Read the model definition and answer for the solid it produces. Units are mm, in the model's axes. Face numbers are marked on the shaded views. A direction names the side the tool comes from. Round coordinates to 2 decimals unless told otherwise and drop trailing zeros. Order: outer loops, then holes, each group sorted by start corner. A loop starts at its lowest first (then second) coordinate and runs counter-clockwise, first axis right, second up. Notation, with made-up numbers: (80, 66.5) - (89, 66.5) arc R20 ccw to (89, 97.5) - close; hole circle Ø11 at (64.5, 70). An arc over 180 degrees is marked (long way). Answer as a JSON object with one key per item and string values. Group by question number.
Q1. Given pin 1 Ø4 at (y, z) = (-4.5, 23) entering from -X; pin 2 Ø1.5 at (y, z) = (-1, -26.5) entering from -X, each flat-ended and moving along its own axis, determine where each tip first touches the part or whether it passes through.
Q2. A cutting plane is placed at C-C on x = -47. Determine the outline of the cut face in (y, z), and give its area (3 significant figures).
Q3. Consider line 1 (X direction, y = -10.5, z = 18.5); line 2 (Z direction, x = -46, y = -1); line 3 (Z direction, x = -42.5, y = -5.5). Determine where each line is inside the solid, lowest interval first.
Q4. The mould has two halves that part along Z. Classify the marked faces 3, 4, 5 and 6: pulls with the +Z half, pulls with the -Z half, needs draft (parallel to the pull), parting line crosses it, or undercut.
Q5. A cutting plane is placed at B-B on y = -10.5. Count the separate pieces of the cut face and the enclosed holes in it, and give its area (3 significant figures).
Q6. A tool of negligible diameter and unlimited length cuts with its end or side. For the marked faces 1 and 2, from which of +Z, -Z, +X, -X, +Y, -Y can it reach the whole face along a straight path? Write none if from no direction.
Q7. A cutting plane is placed at A-A on z = 4. Determine the outline of the cut face in (x, y), and give its area (3 significant figures).
Q8. A cutting plane is placed at D-D on z = 13.5. Determine the outline of the cut face in (x, y).
```python
from build123d import *

# Parameters (mm, degrees)
F0_W     = 115
F0_H     = 70
F1_DEPTH = 12
F2_W     = 4.25
F2_H     = 5
F2_W_2   = 4.2500000007
F3_DEPTH = 25
F4_R     = 3.25
F5_DEPTH = 25
F6_R     = 15


with BuildPart() as f1:
    # F0 (on Front) → F1 (new body)
    with BuildSketch(Plane.XZ):
        Rectangle(F0_W, F0_H)
    extrude(amount=F1_DEPTH)

    # F2 (on face) → F3 (cut)
    with BuildSketch(Plane.XZ.offset(12)):
        with BuildLine():
            Line((-40.75, 16.25), (-40.75, 21.25))
            ThreePointArc((-40.75, 21.25), (-44.9763637107, 25.4999342731), (-49.2497370945, 21.2972718474))
            Line((-49.2497370945, 21.2972718474), (-49.2497419962, 21.2031708885))
            Line((-49.2497419962, 21.2031708885), (-49.2499999942, 16.2502213815))
            ThreePointArc((-49.2499999942, 16.2502213815), (-48.0052820892, 13.2448744512), (-45, 12))
            Line((-45, 12), (-45, 16.25))
            Line((-45, 16.25), (-40.75, 16.25))
        make_face()
        with BuildLine():
            ThreePointArc((49.2497370945, 21.2972718474), (44.9763637107, 25.4999342731), (40.75, 21.25))
            Line((40.75, 21.25), (40.75, 16.25))
            ThreePointArc((40.75, 16.25), (41.99479618, 19.25520382), (45, 20.5))
            ThreePointArc((45, 20.5), (46.9284060776, 20.0373143519), (48.4369317712, 18.75))
            ThreePointArc((48.4369317712, 18.75), (49.041590439, 17.5645519096), (49.2499999942, 16.2502213815))
            Line((49.2499999942, 16.2502213815), (49.2497419962, 21.2031708885))
            Line((49.2497419962, 21.2031708885), (49.2497370945, 21.2972718474))
        make_face()
        with BuildLine():
            ThreePointArc((-45, 12), (-41.99479618, 13.24479618), (-40.75, 16.25))
            Line((-40.75, 16.25), (-45, 16.25))
            Line((-45, 16.25), (-45, 12))
        make_face()
        with BuildLine():
            ThreePointArc((45, 20.5), (41.99479618, 19.25520382), (40.75, 16.25))
            Line((40.75, 16.25), (45, 16.25))
            Line((45, 16.25), (45, 20.5))
        make_face()
        with BuildLine():
            Line((45, 16.25), (40.75, 16.25))
            ThreePointArc((40.75, 16.25), (41.99479618, 13.24479618), (45, 12))
            Line((45, 12), (45, 16.25))
        make_face()
        with BuildLine():
            Line((45, 20.5), (45, 16.25))
            Line((45, 16.25), (45, 12))
            ThreePointArc((45, 12), (48.00520382, 13.24479618), (49.25, 16.25))
            ThreePointArc((49.25, 16.25), (49.2499999986, 16.2501106908), (49.2499999942, 16.2502213815))
            ThreePointArc((49.2499999942, 16.2502213815), (49.041590439, 17.5645519096), (48.4369317712, 18.75))
            ThreePointArc((48.4369317712, 18.75), (46.9284060776, 20.0373143519), (45, 20.5))
        make_face()
        with BuildLine():
            ThreePointArc((-40.75, -16.25), (-41.99479618, -13.24479618), (-45, -12))
            Line((-45, -12), (-45, -16.25))
            Line((-45, -16.25), (-40.75, -16.25))
        make_face()
        with BuildLine():
            Line((-45, -16.25), (-45, -12))
            ThreePointArc((-45, -12), (-48.0052820892, -13.2448744512), (-49.2499999942, -16.2502213815))
            Line((-49.2499999942, -16.2502213815), (-49.2497419962, -21.2031708885))
            Line((-49.2497419962, -21.2031708885), (-49.2497370945, -21.2972718474))
            ThreePointArc((-49.2497370945, -21.2972718474), (-44.9763637107, -25.4999342731), (-40.75, -21.25))
            Line((-40.75, -21.25), (-45, -21.25))
            Line((-45, -21.25), (-45, -16.25))
        make_face()
        with BuildLine():
            ThreePointArc((49.2499999957, -16.2502213815), (48.005242953, -13.2449460071), (45, -12.0001106908))
            Line((45, -12.0001106908), (45, -16.25))
            Line((45, -16.25), (45, -21.25))
            Line((45, -21.25), (40.75, -21.25))
            ThreePointArc((40.75, -21.25), (44.9763637107, -25.4999342731), (49.2497370945, -21.2972718474))
            Line((49.2497370945, -21.2972718474), (49.2497419962, -21.2031708885))
            Line((49.2497419962, -21.2031708885), (49.2499999942, -16.2502213815))
        make_face()
        with BuildLine():
            Line((45, -16.25), (45, -12.0001106908))
            ThreePointArc((45, -12.0001106908), (41.9948353134, -13.2448677349), (40.7499999986, -16.25))
            Line((40.7499999993, -16.25), (45, -16.25))
        make_face()
        with Locations((-42.875, -18.75)):
            Rectangle(F2_W, F2_H)
        with Locations((42.8749999996, -18.75)):
            Rectangle(F2_W_2, F2_H)
    extrude(amount=-F3_DEPTH, mode=Mode.SUBTRACT)

    # F4 (on face) → F5 (cut)
    with BuildSketch(Plane.XZ.offset(12)):
        with Locations((0, 4)):
            Circle(F4_R)
    extrude(amount=-F5_DEPTH, mode=Mode.SUBTRACT)

    # F6
    f6_edges = [f1.edges().sort_by_distance(p)[0] for p in [
        (-57.5, -6, 35),
        (57.5, -6, 35),
        (57.5, -6, -35),
        (-57.5, -6, -35),
    ]]
    fillet(f6_edges, radius=F6_R)


solid = f1.part
```
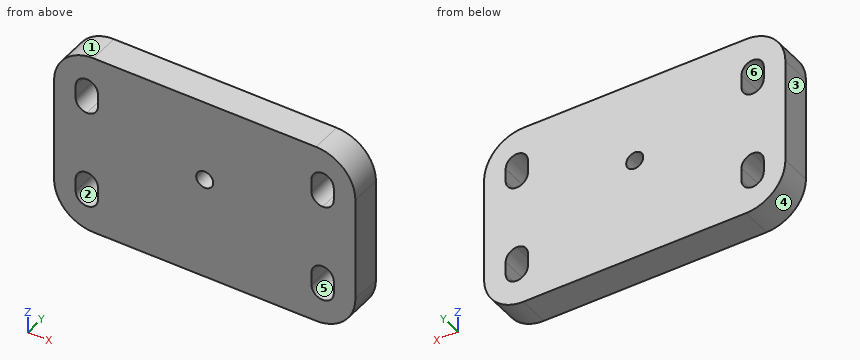
Result set:
{
 "1": {"pin 1": "stops at x = -57.47", "pin 2": "stops at x = -56.35"},
 "2": {"outline": "(-12, -34.31) - (0, -34.31) - (0, -25) - (-12, -25) - close; (-12, -12.5) - (0, -12.5) - (0, 12.5) - (-12, 12.5) - close; (-12, 25) - (0, 25) - (0, 34.31) - (-12, 34.31) - close", "area": "523 mm²"},
 "3": {"line 1": "x = -57.5 to -49.25, -40.75 to 40.75, 49.25 to 57.5", "line 2": "z = -34.59 to -25.38, -12.12 to 12.12, 25.38 to 34.59", "line 3": "z = -35 to -24.69, -12.81 to 12.81, 24.69 to 35"},
 "4": {"face 3": "needs draft", "face 4": "pulls with the -Z half", "face 5": "undercut", "face 6": "undercut"},
 "5": {"separate pieces": "1", "enclosed holes": "5", "area": "7,430 mm²"},
 "6": {"face 1": "+Z, -X, +Y, -Y", "face 2": "+Y, -Y"},
 "7": {"outline": "(-57.5, -12) - (-3.25, -12) - (-3.25, 0) - (-57.5, 0) - close; (3.25, -12) - (57.5, -12) - (57.5, 0) - (3.25, 0) - close", "area": "1,300 mm²"},
 "8": {"outline": "(-57.5, -12) - (-48.24, -12) - (-48.24, 0) - (-57.5, 0) - close; (-41.76, -12) - (41.76, -12) - (41.76, 0) - (-41.76, 0) - close; (48.24, -12) - (57.5, -12) - (57.5, 0) - (48.24, 0) - close"}
}
